CAD build for the part. Positions are in the model's coordinates, mm. Face numbers are marked on the shaded views. A direction names the side the tool comes from. Give positions to 0.01 mm unless a question says otherwise; leave off trailing zeros. Loops run counter-clockwise (first coordinate to the right, second up) from the corner with the lowest first, then second, coordinate; pieces in that order, holes last.
Item 1: Drop flat-ended pins along their axis: P1, Ø3, axis at x = 100, z = 37, coming from the -Y side; P2, Ø6, axis at x = 25, z = 52, coming from the +Y side. Give the stop position or say it passes through.
Item 2: Saw through at D-D on x = 68.5. Give the cut face in (y, z).
Item 3: Saw through at B-B on y = -9.5. Give the cut face in (x, z), plus the area to 3 significant figures.
Item 4: Which spindle directions (+Z, -Z, +X, -X, +Y, -Y) get a long thin tool onto all of the face, cutting with end or side? Do the marked faces 1 and 2. Say none if no direction does.
Item 5: Saw through at A-A on z = 33. Give the cut face in (x, y), plus the area to 3 significant figures.
Item 6: Mould opens along X. For the marked faces 3, 4 and 5 say: released by +X, released by -X, zero draft, split by the parting line, or undercut.
Item 7: Probe probe 1 along X at (y, z) = (-9, 29); probe 2 along Y at (x, z) = (53, 56); probe 3 along Z at (x, y) = (116, -22). List the from-to ranges inside material, lowest first.
Item 8: Saw through at C-C on y = -22.5. Give the cut face in (x, z), plus the area to 3 significant figures.
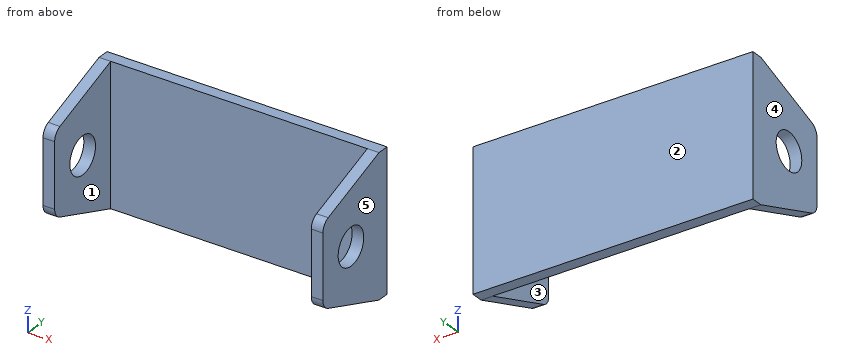
from build123d import *

# Parameters (mm, degrees)
F0_W     = 120
F0_H     = 60
F1_DEPTH = 5
F3_DEPTH = 5
F6_DEPTH = 5
F4_R     = 8
F7_DEPTH = 146
F8_R     = 5


with BuildPart() as f1:
    # F0 (on Front) → F1 (new body)
    with BuildSketch(Plane.XZ):
        with Locations((60, 30)):
            Rectangle(F0_W, F0_H)
    extrude(amount=F1_DEPTH)

    # F2 (on face) → F3 (join)
    with BuildSketch(Plane(origin=(0, 0, 0), x_dir=(0, -1, 0), z_dir=(-1, 0, 0))):
        Polygon((40, 47.261042), (5, 60), (5, 0), (40, 12.738958), align=None)
    extrude(amount=-F3_DEPTH)

    # F5 (on face) → F6 (join)
    with BuildSketch(Plane.YZ.offset(120)):
        Polygon((-5, 0), (-5, 60), (-40, 47.261042), (-40, 12.738958), align=None)
    extrude(amount=-F6_DEPTH)

    # F4 (on face) → F7 (cut)
    with BuildSketch(Plane(origin=(0, 0, 0), x_dir=(0, -1, 0), z_dir=(-1, 0, 0))):
        with Locations((22.5, 29.999479)):
            Circle(F4_R)
    extrude(amount=-F7_DEPTH, mode=Mode.SUBTRACT)

    # F8
    f8_edges = [f1.edges().sort_by_distance(p)[0] for p in [
        (2.5, -40, 47.261042),
        (2.5, -40, 12.738958),
        (117.5, -40, 47.261042),
        (117.5, -40, 12.738958),
    ]]
    fillet(f8_edges, radius=F8_R)


solid = f1.part
Results below:
1. P1: stops at y = -5
1. P2: stops at y = 0
2. outline: (-5, 0) - (0, 0) - (0, 60) - (-5, 60) - close
3. outline: (0, 1.64) - (5, 1.64) - (5, 58.36) - (0, 58.36) - close; (115, 1.64) - (120, 1.64) - (120, 58.36) - (115, 58.36) - close
3. area: 567 mm2
4. face 1: +Z, -Z, -Y
4. face 2: +Z, -Z, +X, -X, +Y
5. outline: (0, -40) - (5, -40) - (5, -29.92) - (0, -29.92) - close; (0, -15.08) - (5, -15.08) - (5, -5) - (115, -5) - (115, -15.08) - (120, -15.08) - (120, 0) - (0, 0) - close; (115, -40) - (120, -40) - (120, -29.92) - (115, -29.92) - close
5. area: 802 mm2
6. face 3: undercut
6. face 4: released by -X
6. face 5: released by +X
7. probe 1: x = 0 to 5, 115 to 120
7. probe 2: y = -5 to 0
7. probe 3: z = 6.19 to 22.02, 37.98 to 53.81
8. outline: (0, 6.37) - (5, 6.37) - (5, 22) - (0, 22) - close; (0, 38) - (5, 38) - (5, 53.63) - (0, 53.63) - close; (115, 6.37) - (120, 6.37) - (120, 22) - (115, 22) - close; (115, 38) - (120, 38) - (120, 53.63) - (115, 53.63) - close
8. area: 313 mm2
